from build123d import *

# Parameters (mm, degrees)
BOSS_EXTRUDE1_DEPTH = 3
FILLET1_R           = 2
SKETCH4_R           = 1.525
SKETCH4_W           = 3
SKETCH4_H           = 5
CUT_EXTRUDE1_DEPTH  = 23.005681085


with BuildPart() as part:
    # Sketch1 → Boss-Extrude1 (new body)
    with BuildSketch(Plane.XY):
        Polygon((-11.5, -10), (-2.5, -10), (-2.5, -13), (2.5, -13), (2.5, -10), (11.5, -10), (11.5, -13), (16.5, -13), (16.5, -10), (17.5, -10), (17.5, 10), (-17.5, 10), (-17.5, -10), (-16.5, -10), (-16.5, -13), (-11.5, -13), align=None)
    extrude(amount=BOSS_EXTRUDE1_DEPTH)

    # Fillet1
    fillet1_edges = [part.edges().sort_by_distance(p)[0] for p in [
        (-17.5, 10, 1.5),
        (17.5, 10, 1.5),
    ]]
    fillet(fillet1_edges, radius=FILLET1_R)

    # Sketch4 → Cut-Extrude1 (cut, through all)
    with BuildSketch(Plane.XY.offset(3)):
        with Locations((-0.68, -0.05)):
            Circle(SKETCH4_R)
        with Locations((-15, -4.5)):
            Rectangle(SKETCH4_W, SKETCH4_H)
        with Locations((15, -4.5)):
            Rectangle(SKETCH4_W, SKETCH4_H)
    extrude(amount=-CUT_EXTRUDE1_DEPTH, mode=Mode.SUBTRACT)


solid = part.part
Geometry: final body of the model. Coordinates: model frame, mm. A direction names the side the tool comes from. Coordinates: 2 decimals unless noted, no trailing zeros. Loops run counter-clockwise (first coordinate to the right, second up) from the corner with the lowest first, then second, coordinate; pieces in that order, holes last. Notation, with made-up numbers: (-34, -11) - (4, -11) arc R29 ccw to (4, 25) - close; hole circle Ø6 at (36, -6). An arc over 180 degrees is marked (long way). Put each result on its own line as item: value. Start each with the question number.
Q1. Set-up query: faces 1 (the flat face through (-16.5, -5, 2)), 2 (the flat face through (11.5, -11, 1)), 3 (the flat face through (-16.5, -11, 1)), 4 (the flat face through (17, -10, 1)). Return all of +Z, -Z, +X, -X, +Y, -Y with unobstructed straight access to the full face (end or side cutting, diameter ignored); none if empty.
Q2. Pin query (flat end, axial travel): pin 1 Ø0.8 at (x, z) = (-17, 2) entering from -Y; pin 2 Ø1.5 at (y, z) = (-12, 1) entering from -X; pin 3 Ø0.9 at (y, z) = (-11, 1) entering from +X. Return the tip coordinate at first contact, or that it passes through.
Q3. Pull-direction query (X, two-part tool) for faces 5 (the cylindrical face through (16.93, 9.4, 1.52)), 6 (the flat face through (7, -10, 1)), 7 (the flat face through (0, 10, 1)), 8 (the flat face through (-15, -7, 2)); classes: released by +X, released by -X, zero draft, split by the parting line, or undercut.
Q4. Cut plane A-A, the plane y = -0.05. Return loops of the section in (x, z) (3 decimals).
Q5. Cut plane B-B, the plane x = -0.68. Return loops of the section in (y, z) (3 decimals), and give its area (4 significant figures).
Q6. Line query: line 1 (Y direction, x = -0.68, z = 1.55) (3 decimals); line 2 (Y direction, x = -15, z = 1.25); line 3 (Y direction, x = 5, z = 2.6). Output: solid intervals per line, ascending.
Q7. Cut plane C-C, the plane z = 1.9. Return loops of the section in (x, y) (3 decimals), and give its area (3 significant figures).
Q8. Cut plane D-D, the plane x = 8. Return loops of the section in (y, z), and give its area (3 significant figures).
Filled sheet:
1. face 1: +Z, -Z
1. face 2: +Z, -Z, -Y
1. face 3: +Z, -Z, -X, -Y
1. face 4: +Z, -Z, +X, -Y
2. pin 1: y = -10
2. pin 2: x = -16.5
2. pin 3: x = 16.5
3. face 5: released by +X
3. face 6: undercut
3. face 7: zero draft
3. face 8: undercut
4. outline: (-17.5, 0) - (-2.205, 0) - (-2.205, 3) - (-17.5, 3) - close; (0.845, 0) - (17.5, 0) - (17.5, 3) - (0.845, 3) - close
5. outline: (-13, 0) - (-1.575, 0) - (-1.575, 3) - (-13, 3) - close; (1.475, 0) - (10, 0) - (10, 3) - (1.475, 3) - close
5. area: 59.85 mm²
6. line 1: -13 to -1.575, 1.475 to 10
6. line 2: -13 to -7, -2 to 10
6. line 3: -10 to 10
7. outline: (-17.5, -10) - (-16.5, -10) - (-16.5, -13) - (-11.5, -13) - (-11.5, -10) - (-2.5, -10) - (-2.5, -13) - (2.5, -13) - (2.5, -10) - (11.5, -10) - (11.5, -13) - (16.5, -13) - (16.5, -10) - (17.5, -10) - (17.5, 8) arc R2 ccw to (15.5, 10) - (-15.5, 10) arc R2 ccw to (-17.5, 8) - close; hole (-16.5, -7) - (-13.5, -7) - (-13.5, -2) - (-16.5, -2) - close; hole circle Ø3.05 at (-0.68, -0.05); hole (13.5, -7) - (16.5, -7) - (16.5, -2) - (13.5, -2) - close
7. area: 706 mm²
8. outline: (-10, 0) - (10, 0) - (10, 3) - (-10, 3) - close
8. area: 60.0 mm²
